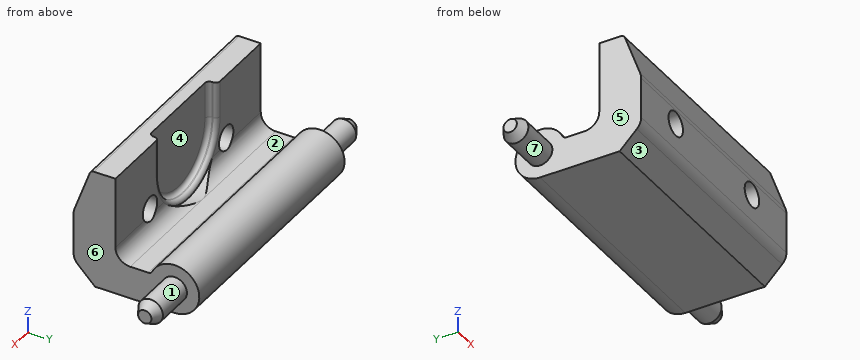
Autodesk Inventor part; units mm, degrees
ref_plane "DECKEL_XY" through (0, 10.25, -3) normal (1, 0, 0) x (0, 0, -1)
ref_plane "DECKEL_YZ" through (0, 10.25, -3) normal (0, 0, -1) x (0, 1, 0)
ref_plane "DECKEL_ZX" through (0, 10.25, -3) normal (0, 1, 0) x (1, 0, 0)
sketch "Sketch_1" plane through (0, 0, 0) normal (1, 0, 0) x (0, 0, -1)
  line L0 (-6.5, 4.25) -> (-6.5, 2.0679)
  arc A0 (-6.5, 2.0679) -> (-6.2039, 1.645) centre (-6.05, 2.0679) ccw
  line L1 (-6.2039, 1.645) -> (-1.9329, 0.0905)
  arc A1 (-1.9329, 0.0905) -> (-1.4198, 0) centre (-1.4198, 1.5) ccw
  line L2 (-1.4198, 0) -> (2.6944, 0)
  arc A2 (2.6944, 0) -> (3.755, 0.4393) centre (2.6944, 1.5) ccw
  line L3 (3.755, 0.4393) -> (5.5, 2.1843)
  line L4 (5.5, 2.1843) -> (5.5, 10.25)
  arc A3 (5.5, 10.25) -> (1.9407, 7.9855) centre (3, 10.25) ccw
  arc A4 (2.2, 7.5779) -> (1.9407, 7.9855) centre (1.75, 7.5779) ccw
  line L5 (2.2, 7.5779) -> (2.2, 5.75)
  arc A5 (0.7, 4.25) -> (2.2, 5.75) centre (0.7, 5.75) ccw
  line L6 (0.7, 4.25) -> (-6.5, 4.25)
extrude "Extrusion1" add sketch "Sketch_1" along normal mid plane 24.8
sketch "Sketch2" plane through (-12.4, 0, -2.6944) normal (0, -1, 0) x (1, 0, 0)
  point P0 (18.9, 2.6944)
hole "Hole1" at (6.5, 0, 0) direction (0, 1, 0) diameter 2.459 depth 5.75
sketch "Sketch3" plane through (-12.4, 0, -2.6944) normal (0, -1, 0) x (1, 0, 0)
  point P0 (5.9, 2.6944)
hole "Hole2" at (-6.5, 0, 0) direction (0, 1, 0) diameter 2.459 depth 5.75
sketch "Sketch_5" plane through (0, 0, 6.5) normal (0, 0, 1) x (1, 0, 0)
  arc A0 (-5, 3.8) -> (-5.45, 4.25) centre (-5.45, 3.8) ccw
  line L0 (-5, 3.8) -> (-5, 3.7)
  arc A1 (-5, 3.7) -> (-4.55, 3.25) centre (-4.55, 3.7) ccw
  line L1 (-4.55, 3.25) -> (4.55, 3.25)
  arc A2 (4.55, 3.25) -> (5, 3.7) centre (4.55, 3.7) ccw
  line L2 (5, 3.7) -> (5, 3.8)
  arc A3 (5.45, 4.25) -> (5, 3.8) centre (5.45, 3.8) ccw
  line L3 (5.45, 4.25) -> (5.45, 7.25)
  line L4 (5.45, 7.25) -> (-5.45, 7.25)
  line L5 (-5.45, 7.25) -> (-5.45, 4.25)
extrude "Extrusion2" cut sketch "Sketch_5" against normal blind 3.7
sketch "Sketch_6" plane through (0, 0, 2.8) normal (0, 0, 1) x (1, 0, 0)
  line L0 (0, 3.25) -> (0, 7.25)
  line L1 (0, 7.25) -> (4.55, 7.25)
  line L2 (4.55, 7.25) -> (5.45, 4.25)
  arc A0 (5.45, 4.25) -> (5, 3.8) centre (5.45, 3.8) ccw
  line L3 (5, 3.8) -> (5, 3.7)
  arc A1 (4.55, 3.25) -> (5, 3.7) centre (4.55, 3.7) ccw
  line L4 (4.55, 3.25) -> (0, 3.25)
  line L5 (0, 3.25) -> (0, 7.25)
revolve "Revolution1" cut sketch "Sketch_6" angle 180 about axis through (0, 3.25, 2.8) along (0, 1, 0)
sketch "Sketch_8" plane through (0, 0, -3) normal (0, 0, 1) x (1, 0, 0)
  line L0 (17.5, 10.25) -> (-17.5, 10.25)
  line L1 (-17.5, 10.25) -> (-17.5, 10.925)
  line L2 (-17.5, 10.925) -> (-16.5, 11.5)
  line L3 (-16.5, 11.5) -> (16.5, 11.5)
  line L4 (16.5, 11.5) -> (17.5, 10.925)
  line L5 (17.5, 10.925) -> (17.5, 10.25)
  line L6 (17.5, 10.25) -> (-17.5, 10.25)
revolve "Revolution2" add sketch "Sketch_8" angle 360 about axis through (17.5, 10.25, -3) along (1, 0, 0)
ref_plane "DECKEL_XY" through (0, 10.25, -3) normal (1, 0, 0) x (0, 0, -1)
ref_plane "DECKEL_YZ" through (0, 10.25, -3) normal (0, 0, -1) x (0, 1, 0)
ref_plane "DECKEL_ZX" through (0, 10.25, -3) normal (0, 1, 0) x (1, 0, 0)
ref_plane "HINGE_XY" through (0, 0, 0) normal (1, 0, 0) x (0, 0, -1)
ref_plane "HINGE_YZ" through (0, 0, 0) normal (0, 0, -1) x (0, 1, 0)
ref_plane "HINGE_ZX" through (0, 0, 0) normal (0, 1, 0) x (1, 0, 0)
properties part number "1301.000_4_(1)"
For this review, take the finished solid that the model builds, in its own axes (mm). Face numbers are marked on the shaded views. A direction names the side the tool comes from. Give positions to 0.01 mm unless a question says otherwise; leave off trailing zeros. Loops run counter-clockwise (first coordinate to the right, second up) from the corner with the lowest first, then second, coordinate; pieces in that order, holes last. Notation, with made-up numbers: M -14,16.25 L 39,16.25 A32 ccw 39,46.25 Z; hole C 3.25,13.25 d7. An arc over 180 degrees is marked long. One line per item, written item: value. Start each with the question number.
Q1. Add section B-B (y = 1.25). Give the boundary of the cut face in (x, z), and give its area (3 significant figures).
Q2. Clearance check with flat-ended pins moving along their axes: pin 1 Ø1 at (x, z) = (-1, -2) entering from +Y; pin 2 Ø1 at (x, z) = (12.5, 2.5) entering from +Y; pin 3 Ø1.5 at (x, z) = (-5, -1) entering from -Y; pin 4 Ø2 at (x, z) = (-6.5, 0) entering from -Y. State where each tip first meets the part, or that it passes through.
Q3. For L1, parallel to X at y = 2.3, z = 0; L2, parallel to Z at x = 6.5, y = 3.55; L3, parallel to Y at x = -10, z = 0.25, list the stretches that pass through material, from the lowest coordinate up.
Q4. Add section D-D (z = 4). Give the boundary of the cut face in (x, y).
Q5. Machinability: for the marked faces 1, 2 and 3, which of the approach directions +Z, -Z, +X, -X, +Y, -Y give a long, thin tool a straight path to every point of the face, cutting with its end or side? Answer none if there is none.
Q6. Draft analysis for pull direction X (two halves, no side actions). For the marked faces 4, 5, 6 and 7, state which applies: released by +X, released by -X, zero draft, split by the parting line, or undercut.
Reply:
1. outline: M -12.4,-4.57 L 12.4,-4.57 L 12.4,5.12 L -12.4,5.12 Z; hole C -6.5,0 d2.46; hole C 6.5,0 d2.46
1. area: 231 mm²
2. pin 1: y = 12.7
2. pin 2: y = 4.25
2. pin 3: y = 0
2. pin 4: y = 8.75
3. L1: -12.4 to -7.73, -5.27 to 5.27, 7.73 to 12.4
3. L2: -5.5 to -1.23, 1.23 to 6.5
3. L3: 0 to 4.25
4. outline: M -12.4,0.84 L 12.4,0.84 L 12.4,4.25 L 5.45,4.25 A0.45 ccw 5,3.8 L 5,3.7 A0.45 cw 4.55,3.25 L -4.55,3.25 A0.45 cw -5,3.7 L -5,3.8 A0.45 ccw -5.45,4.25 L -12.4,4.25 Z
5. face 1: +X
5. face 2: +Z, +X, -X
5. face 3: -Z, +X, -X, -Y
6. face 4: undercut
6. face 5: released by -X
6. face 6: released by +X
6. face 7: zero draft
